Here's how the part is built. I have some questions about the finished solid (model axes, mm). A direction names the side the tool comes from. Round coordinates to 2 decimals unless told otherwise and drop trailing zeros. Order: outer loops, then holes, each group sorted by start corner. A loop starts at its lowest first (then second) coordinate and runs counter-clockwise, first axis right, second up. Notation, with made-up numbers: (-38.75, 77.25) - (1.25, 77.25) arc R25 ccw to (1.25, 89.25) - close; hole circle Ø8 at (37, 2.25). An arc over 180 degrees is marked (long way). One line per item, written item: value.
from build123d import *

# Parameters (mm, degrees)
F0_R      = 3.175
F1_DEPTH  = 11.43
F5_DEPTH  = 25.4
F6_D      = 6.35
F6_DEPTH  = 76.2
F6_TIP    = 1.9077324654
F7_D      = 6.35
F7_DEPTH  = 76.2
F7_TIP    = 1.9077324654
F8_D      = 6.35
F8_DEPTH  = 76.2
F8_TIP    = 1.9077324654
F9_D      = 6.35
F9_DEPTH  = 76.2
F9_TIP    = 1.9077324654
F11_DEPTH = 95.25


with BuildPart() as f1:
    # F0 (on Right) → F1 (new body)
    with BuildSketch(Plane.YZ):
        Polygon((122.1165703362, -43.8827651219), (122.1165703362, 51.3672348781), (-90.1177801321, 90.9827682114), (-67.7204277456, -59.7624426779), align=None)
        with Locations((109.9245703362, -34.0493256675)):
            Circle(F0_R, mode=Mode.SUBTRACT)
        with Locations((109.9245703362, 20.0526743325)):
            Circle(F0_R, mode=Mode.SUBTRACT)
        with Locations((90.3665703362, 36.3643222504)):
            Circle(F0_R, mode=Mode.SUBTRACT)
        with Locations((90.3665703362, 36.3643222504)):
            Circle(F0_R)
        with Locations((109.9245703362, 20.0526743325)):
            Circle(F0_R)
        with Locations((109.9245703362, -34.0493256675)):
            Circle(F0_R)
    extrude(amount=F1_DEPTH)


with BuildPart() as f1_1:
    # F2: moved
    add(f1.part.moved(Location((47.625, 0, 0))))


with BuildPart() as f3_1:
    # F3: instance of F1
    add(f1_1.part.mirror(Plane.YZ))

    # F4 (on face) → F5 (cut)
    with BuildSketch(Plane(origin=(-59.055, 0, 0), x_dir=(0, -1, 0), z_dir=(-1, 0, 0))):
        with BuildLine():
            ThreePointArc((17.5834296638, -43.8827651219), (-33.2165703362, 6.9172348781), (-84.0165703362, -43.8827651219))
            ThreePointArc((-84.0165703362, -43.8827651219), (-83.9914140751, -45.4812779607), (-83.9159702065, -47.0782076259))
            Line((-83.9159702065, -47.0782076259), (16.2473795848, -55.4567729935))
            ThreePointArc((16.2473795848, -55.4567729935), (17.2483117898, -49.7081983252), (17.5834296638, -43.8827651219))
        make_face()
        with BuildLine():
            Line((17.5834296638, -55.5685322642), (17.5834296638, -43.8827651219))
            ThreePointArc((17.5834296638, -43.8827651219), (17.2483117898, -49.7081983252), (16.2473795848, -55.4567729935))
            Line((16.2473795848, -55.4567729935), (17.5834296638, -55.5685322642))
        make_face()
    extrude(amount=-F5_DEPTH, mode=Mode.SUBTRACT)

    # F6
    with Locations(Plane.YZ):
        with Locations((90.3665703362, 36.3643222504)):
            Hole(F6_D / 2, depth=F6_DEPTH)
            with Locations((0, 0, -(F6_DEPTH + F6_TIP / 2))):  # 118° drill point
                Cone(0, F6_D / 2, F6_TIP, mode=Mode.SUBTRACT)

    # F7
    with Locations(Plane.YZ):
        with Locations((109.9245703362, 20.0526743325)):
            Hole(F7_D / 2, depth=F7_DEPTH)
            with Locations((0, 0, -(F7_DEPTH + F7_TIP / 2))):  # 118° drill point
                Cone(0, F7_D / 2, F7_TIP, mode=Mode.SUBTRACT)

    # F8
    with Locations(Plane.YZ):
        with Locations((109.9245703362, -34.0493256675)):
            Hole(F8_D / 2, depth=F8_DEPTH)
            with Locations((0, 0, -(F8_DEPTH + F8_TIP / 2))):  # 118° drill point
                Cone(0, F8_D / 2, F8_TIP, mode=Mode.SUBTRACT)


with BuildPart() as f1_2:
    add(f1_1.part)

    # F9
    with Locations(Plane(origin=(0, 0, 0), x_dir=(0, 1, 0), z_dir=(-1, 0, 0))):
        with Locations((90.3665703362, -36.3643222504)):
            Hole(F9_D / 2, depth=F9_DEPTH)
            with Locations((0, 0, -(F9_DEPTH + F9_TIP / 2))):  # 118° drill point
                Cone(0, F9_D / 2, F9_TIP, mode=Mode.SUBTRACT)


with BuildPart() as f11:
    # F10 (on face) → F11 (new body)
    with BuildSketch(Plane(origin=(47.625, 0, 0), x_dir=(0, -1, 0), z_dir=(-1, 0, 0))):
        with BuildLine():
            Line((46.0226261079, 141.3909337274), (55.0595276774, 113.1756901692))
            ThreePointArc((55.0595276774, 113.1756901692), (61.2467442889, 100.0992346093), (66.2609327925, 86.5296637591))
            Line((66.2609327925, 86.5296637591), (48.4415836851, 142.1656880364))
            Line((48.4415836851, 142.1656880364), (46.0226261079, 141.3909337274))
        make_face()
        with BuildLine():
            Line((55.0595276774, 113.1756901692), (63.7442887749, 86.0599085345))
            Line((63.7442887749, 86.0599085345), (66.2609327925, 86.5296637591))
            ThreePointArc((66.2609327925, 86.5296637591), (61.2467442889, 100.0992346093), (55.0595276774, 113.1756901692))
        make_face()
        with BuildLine():
            Line((63.7442887749, 86.0599085345), (63.7439748969, 86.0598499462))
            ThreePointArc((63.7439748969, 86.0598499462), (69.5928864987, 61.5174094181), (71.5584296638, 36.3643222504))
            ThreePointArc((71.5584296638, 36.3643222504), (66.8411203346, -2.4357759317), (52.9640480804, -38.9751723676))
            Line((52.9640480804, -38.9751723676), (55.2290606215, -40.1252095237))
            ThreePointArc((55.2290606215, -40.1252095237), (69.3114207434, -3.0269888444), (74.0984296638, 36.3643222504))
            ThreePointArc((74.0984296638, 36.3643222504), (72.1272426646, 61.7512669557), (66.2609327925, 86.5296637591))
            Line((66.2609327925, 86.5296637591), (63.7442887749, 86.0599085345))
        make_face()
    extrude(amount=F11_DEPTH)


solid = f3_1.part
Q1. If we section it at A-A, the plane z = 0: Please give me the cut outline in (x, y) (3 decimals).
Results list:
outline: (-59.055, -76.6) - (-47.625, -76.6) - (-47.625, 7.625) - (-59.055, 7.625) - close; (-59.055, 58.808) - (-47.625, 58.808) - (-47.625, 122.117) - (-59.055, 122.117) - close
Q2. If we section it at D-D, the plane z = -41: Please give me the cut outline in (x, y) (3 decimals), then the cut area to 3 significant figures.
Results list:
outline: (-59.055, -70.508) - (-47.625, -70.508) - (-47.625, -17.502) - (-59.055, -17.502) - close; (-59.055, 83.935) - (-47.625, 83.935) - (-47.625, 122.117) - (-59.055, 122.117) - close
area: 1,040 mm²
Q3. We'd pull the mould along Z, two halves only. Please class faces 3 (the flat face through (-53, 122.117, 3)), 4 (the flat face through (-53.26, 17.485, 70.898)), 5 (the cylindrical face through (-53.42, 90.78, 39.512)), 6 (the flat face through (-53.26, -79.076, 16.665)): released by +Z, released by -Z, zero draft, split by the parting line, or undercut.
Results list:
face 3: zero draft
face 4: released by +Z
face 5: undercut
face 6: released by -Z
Q4. If we section it at B-B, the plane x = -50: Please give me the cut outline in (y, z) (3 decimals).
Results list:
outline: (-90.118, 90.983) - (-67.72, -59.762) - (-17.583, -55.569) - (-17.583, -43.883) arc R50.8 cw (long way) to (83.916, -47.078) - (122.117, -43.883) - (122.117, 51.367) - close; hole circle Ø6.35 at (90.367, 36.364); hole circle Ø6.35 at (109.925, -34.049); hole circle Ø6.35 at (109.925, 20.053)
Q5. If we section it at C-C, the plane y = -24: Please give me the cut outline in (x, z) (3 decimals), then the cut area to 3 significant figures.
Results list:
outline: (-59.055, -56.105) - (-47.625, -56.105) - (-47.625, 78.641) - (-59.055, 78.641) - close
area: 1,540 mm²
Q6. Will these pins go through, and if not, where does the flat tip stop? pin 1 (3 mm diameter, centred on x = -50, y = 60.5, fed in from +Z); pin 2 (4 mm diameter, centred on x = -57, z = -16.5, fed in from -Y); pin 3 (10 mm diameter, centred on y = 109.92, z = -34.05, fed in from +X) (3 decimals); pin 4 (5 mm diameter, centred on x = -53.5, z = -33.5, fed in from -Y).
Results list:
pin 1: z = 63.15
pin 2: y = -74.45
pin 3: x = -47.625
pin 4: y = -71.99
Q7. Which directions (+Z, -Z, +X, -X, +Y, -Y) give clear straight access to the entire face, cutting with the end or side of a thin tool? Please do faces 1 (the flat face through (-53, -17.583, -50)), 2 (the flat face through (-47.625, 15, 17)).
Results list:
face 1: -Z, +X, -X
face 2: +Z, -Z, +X, +Y, -Y
Q8. If I drill on line 1 along Y through (x, z) = (-54, -1.5); line 2 along Z through (x, y) = (-56.5, 92.5); line 3 along Y through (x, z) = (-51.75, -30), over which ranges is the centre line in solid material (lowest first)?
Results list:
line 1: -76.38 to 5.21, 61.22 to 122.12
line 2: -46.36 to 34.01, 38.72 to 56.9
line 3: -72.14 to -15.65, 82.08 to 122.12
